Work out the finished part from the listing and answer in its coordinate system (mm). Coordinates: 2 decimals unless noted, no trailing zeros. Write each loop counter-clockwise with the first axis right and the second up, starting at its lowest first coordinate (ties: lowest second). Pieces come first, ordered by that corner, then holes. Notation, with made-up numbers: (15, 77.5) - (31, 77.5) arc R19 cw to (31, 113.5) - close; hole circle Ø10 at (9, -11.5). An arc over 180 degrees is marked (long way). One line per item, written item: value.
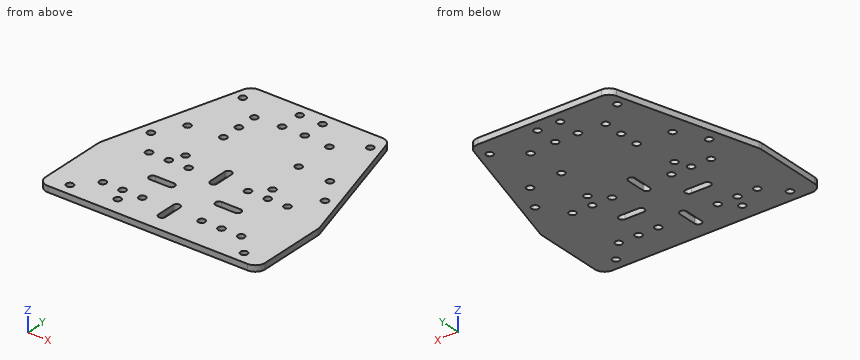
```python
from build123d import *

# Parameters (mm, degrees)
EXTRUDE_1_DEPTH         = 3
HOLE_WIZARD_3_5_3_5_1_D = 3.5
CUT_EXTRUDE_1_DEPTH     = 4
FILLET_1_R              = 5


with BuildPart() as part:
    # 草图1 → 凸台-拉伸1 (new body)
    with BuildSketch(Plane.XY):
        Polygon((-55.5, 0), (-55.5, -40), (55.5, -40), (55.5, 0), (35, 72), (-35, 72), align=None)
    extrude(amount=EXTRUDE_1_DEPTH)

    # Ø3.5 (3.5) 直径孔1 (through all)
    with Locations(Plane.XY.offset(3)):
        with Locations((-5.75, 54.5), (5.75, 54.5), (5.75, 66), (-5.75, 66), (-32.25, 63), (-36, 32), (36, 32), (32.25, 63), (-44, 18.5), (44, 18.5), (44, -34), (-44, -34), (-22, -31.25), (-15, -24.25), (15, -24.25), (15, 5.75), (-15, 5.75), (-22, 12.75), (22, 12.75), (-19, 53.5), (-19, 43.5), (-19, 33.5), (19, 33.5), (19, 53.5), (-25, 5.75), (-25, -24.25), (-35, 5.75), (-35, -24.25), (25, 5.75), (35, 5.75), (35, -24.25), (25, -24.25)):
            Hole(HOLE_WIZARD_3_5_3_5_1_D / 2)

    # 草图2 → 切除-拉伸1 (cut, through all)
    with BuildSketch(Plane.XY.offset(3)):
        with BuildLine():
            Line((1.75, -21.25), (1.75, -30.75))
            ThreePointArc((1.75, -30.75), (0, -32.5), (-1.75, -30.75))
            Line((-1.75, -30.75), (-1.75, -21.25))
            ThreePointArc((-1.75, -21.25), (0, -19.5), (1.75, -21.25))
        make_face()
        with BuildLine():
            Line((12, -7.5), (21.5, -7.5))
            ThreePointArc((21.5, -7.5), (23.25, -9.25), (21.5, -11))
            Line((21.5, -11), (12, -11))
            ThreePointArc((12, -11), (10.25, -9.25), (12, -7.5))
        make_face()
        with BuildLine():
            Line((1.75, 2.75), (1.75, 12.25))
            ThreePointArc((1.75, 12.25), (0, 14), (-1.75, 12.25))
            Line((-1.75, 12.25), (-1.75, 2.75))
            ThreePointArc((-1.75, 2.75), (0, 1), (1.75, 2.75))
        make_face()
        with BuildLine():
            Line((-12, -7.5), (-21.5, -7.5))
            ThreePointArc((-21.5, -7.5), (-23.25, -9.25), (-21.5, -11))
            Line((-21.5, -11), (-12, -11))
            ThreePointArc((-12, -11), (-10.25, -9.25), (-12, -7.5))
        make_face()
    extrude(amount=-CUT_EXTRUDE_1_DEPTH, mode=Mode.SUBTRACT)

    # 圆角1
    fillet_1_edges = [part.edges().sort_by_distance(p)[0] for p in [
        (55.5, 0, 1.5),
        (55.5, -40, 1.5),
        (-55.5, -40, 1.5),
        (-55.5, 0, 1.5),
        (-35, 72, 1.5),
        (35, 72, 1.5),
    ]]
    fillet(fillet_1_edges, radius=FILLET_1_R)


solid = part.part
```
Item 1: Section A-A, the plane x = -5.75 is taken. Determine the outline of the cut face in (y, z).
Evaluation:
outline: (-40, 0) - (52.75, 0) - (52.75, 3) - (-40, 3) - close; (56.25, 0) - (64.25, 0) - (64.25, 3) - (56.25, 3) - close; (67.75, 0) - (72, 0) - (72, 3) - (67.75, 3) - close
Item 2: Consider probe 1 along Y at (x, z) = (-19, 0.9); probe 2 along Y at (x, z) = (-15, 2); probe 3 along Y at (x, z) = (17, 0.25). Determine where each line is inside the solid, lowest interval first.
Evaluation:
probe 1: y = -40 to -11, -7.5 to 31.75, 35.25 to 41.75, 45.25 to 51.75, 55.25 to 72
probe 2: y = -40 to -26, -22.5 to -11, -7.5 to 4, 7.5 to 72
probe 3: y = -40 to -11, -7.5 to 72
Item 3: Given pin 1 (4.5 mm diameter, centred on x = -19, y = 43.5, fed in from -Z); pin 2 (0.9 mm diameter, centred on y = 6, z = 1, fed in from +X), each flat-ended and moving along its own axis, determine where each tip first touches the part or whether it passes through.
Evaluation:
pin 1: stops at z = 0
pin 2: stops at x = 53.92
Item 4: Section B-B, the plane y = -24.25 is taken. Give the number of separate pieces and of enclosed holes in the cut face, then the cut area to 4 significant figures.
Evaluation:
separate pieces: 8
enclosed holes: 0
area: 259.5 mm2
